The drawing under review shows one solid part. Ordinate dimensions are in mm from its lowest x, y, z. Give positions to 0.01 mm unless a question says otherwise; leave off trailing zeros. Order: outer loops, then holes, each group sorted by start corner. A loop starts at its lowest first (then second) coordinate and runs counter-clockwise, first axis right, second up. Notation, with made-up numbers: (-35.75, 66) -> (23.25, 66) arc R17 ccw to (23.25, 94) -> close; hole circle Ø11 at (-9, 2.5). An arc over 180 degrees is marked (long way). Return JSON: item names as keys, results as strings. Group by question number.
1) The part is to be moulded in two halves that separate along Z. For the marked faces 1, 2 and 3, say which applies: released by +Z, released by -Z, zero draft, split by the parting line, or undercut.
2) Add section B-B (y = 45.5). Give the boundary of the cut face in (x, z).
3) Insertion check: P1, Ø10, axis at y = 11.5, z = 56, coming from the +X side; P2, Ø2, axis at y = 10.5, z = 84, coming from the +X side; P3, Ø10, axis at y = 33, z = 81.5, coming from the +X side; P4, Ø5.5, axis at x = 49, z = 49, coming from the -Y side. Each pin has a flat end and moves straight along its axis. Give the tip position at first contact, or say it passes through.
4) To check wall thickness, follow line 1 along Z through (x, y) = (49, 36); line 2 along X through (y, z) = (10.5, 50); line 3 along X through (y, z) = (43.5, 29). State the ranges of each line that lie inside material, in increasing order.
5) Add section A-A (y = 33). Give the boundary of the cut face in (x, z), then the cut area to 3 significant figures.
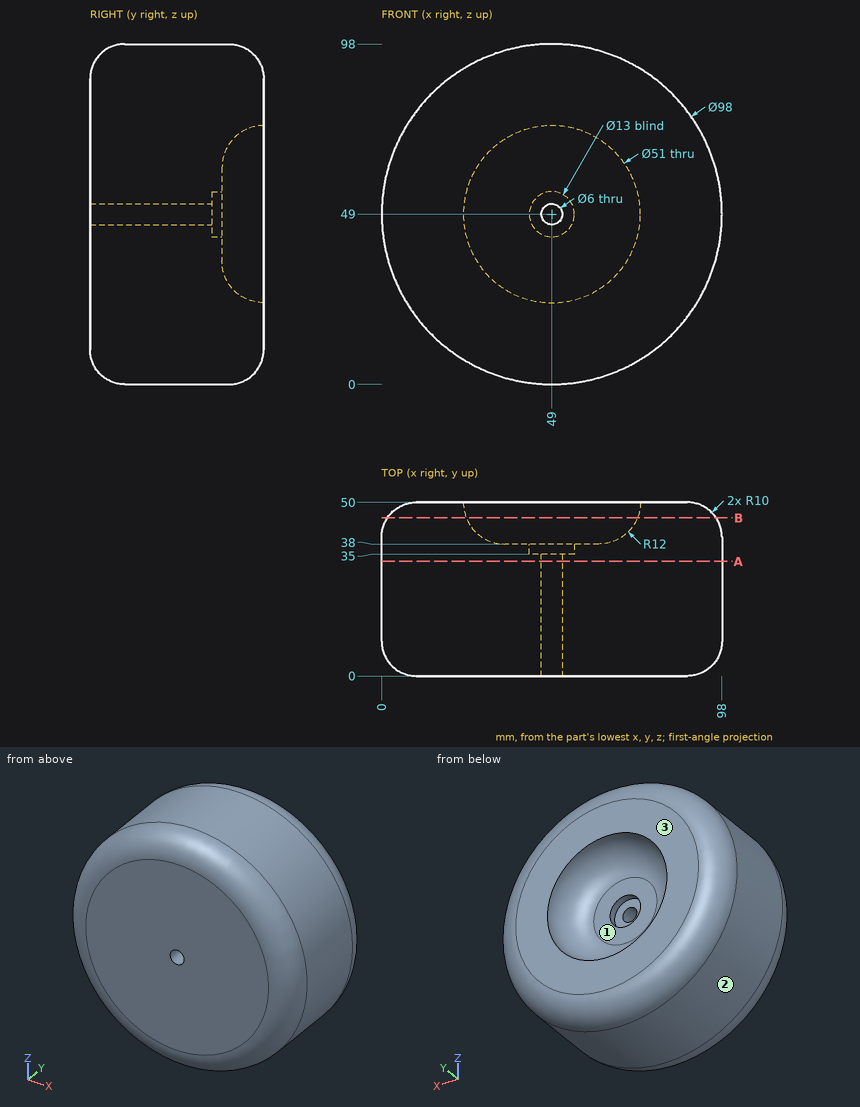
Evaluation:
{
 "1": {"face 1": "undercut", "face 2": "split by the parting line", "face 3": "zero draft"},
 "2": {"outline": "circle Ø94.7 at (49, 49); hole circle Ø49.25 at (49, 49)"},
 "3": {"P1": "x = 97.96", "P2": "x = 84.28", "P3": "x = 89.56", "P4": "through"},
 "4": {"line 1": "0 to 42.5, 55.5 to 98", "line 2": "0.01 to 46.17, 51.83 to 97.99", "line 3": "4.96 to 36.5, 61.5 to 93.04"},
 "5": {"outline": "circle Ø98 at (49, 49); hole circle Ø6 at (49, 49)", "area": "7,510 mm^2"}
}
